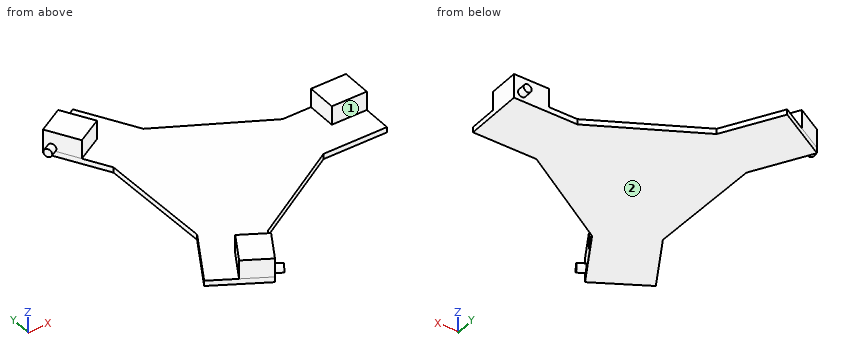
```python
from build123d import *

# Parameters (mm, degrees)
BOSS_EXTRUDE1_DEPTH = 2
SKETCH2_W           = 6.854235104
SKETCH2_H           = 13.064732657
BOSS_EXTRUDE2_DEPTH = 11
SKETCH3_W           = 13.064732657
SKETCH3_H           = 11
BOSS_EXTRUDE3_DEPTH = 7
SKETCH6_R           = 1.5
BOSS_EXTRUDE4_DEPTH = 3
SKETCH7_R           = 1.5
BOSS_EXTRUDE5_DEPTH = 3
SKETCH8_R           = 1.5
BOSS_EXTRUDE6_DEPTH = 3


with BuildPart() as part:
    # Sketch1 → Boss-Extrude1 (new body)
    with BuildSketch(Plane.XY):
        Polygon((30.93899215, 11.451445147), (54.645492629, 11.451445147), (54.645492629, -10.246029868), (30.93899215, -10.246029868), (-5.552253668, -32.519675743), (-17.405503908, -53.050107393), (-36.196068468, -42.201369885), (-24.342818229, -21.670938236), (-25.386738482, 21.068230596), (-37.239988722, 41.598662246), (-18.449424161, 52.447399753), (-6.596173922, 31.916968104), align=None)
    extrude(amount=BOSS_EXTRUDE1_DEPTH)

    # Sketch2 → Boss-Extrude2 (add)
    with BuildSketch(Plane(origin=(-9.917242407, -5.725722573, 0), x_dir=(0, 0, 1), z_dir=(-0.8660254037844431, -0.4999999999999922, 0))):
        with Locations((5.427117552, 48.1131263)):
            Rectangle(SKETCH2_W, SKETCH2_H)
    extrude(amount=-BOSS_EXTRUDE2_DEPTH)

    # Sketch3 → Boss-Extrude3 (add)
    with BuildSketch(Plane.XY.offset(2)):
        Polygon((-37.239988722, 41.598662246), (-27.71370928, 47.098662246), (-21.181342951, 35.784271871), (-30.707622393, 30.284271871), align=None)
        with Locations((48.1131263, 5.951445147)):
            Rectangle(SKETCH3_W, SKETCH3_H)
        Polygon((-10.873137579, -41.735717017), (-17.405503908, -53.050107393), (-26.931783349, -47.550107393), (-20.39941702, -36.235717017), align=None)
    extrude(amount=BOSS_EXTRUDE3_DEPTH)

    # Sketch6 → Boss-Extrude4 (add)
    with BuildSketch(Plane(origin=(-9.917242407, -5.725722573, 0), x_dir=(0, 0, 1), z_dir=(-0.8660254037844431, -0.4999999999999922, 0))):
        with Locations(Location((3, 51.645492629, 0), (0, 0, 270))):
            Circle(SKETCH6_R)
    extrude(amount=BOSS_EXTRUDE4_DEPTH)

    # Sketch7 → Boss-Extrude5 (add)
    with BuildSketch(Plane(origin=(9.917242407, -5.725722573, 0), x_dir=(0, 0, -1), z_dir=(0.8660254037844364, -0.5000000000000041, 0))):
        with Locations(Location((-3.057556163, -51.645492629, 0), (0, 0, 90))):
            Circle(SKETCH7_R)
    extrude(amount=BOSS_EXTRUDE5_DEPTH)

    # Sketch8 → Boss-Extrude6 (add)
    with BuildSketch(Plane(origin=(0, 11.451445147, 0), x_dir=(1, 0, 0), z_dir=(0, 1, 0))):
        with Locations(Location((51.645492629, -3, 0), (0, 0, 270))):
            Circle(SKETCH8_R)
    extrude(amount=BOSS_EXTRUDE6_DEPTH)


solid = part.part
```
Read the model definition and answer for the solid it produces. Units are mm, in the model's axes. Face numbers are marked on the shaded views. A direction names the side the tool comes from. Give positions to 0.01 mm unless a question says otherwise; leave off trailing zeros. Write each loop counter-clockwise with the first axis right and the second up, starting at its lowest first coordinate (ties: lowest second). Pieces come first, ordered by that corner, then holes. Notation, with made-up numbers: (43, 30) - (67, 30) arc R22 cw to (67, 36) - close; hole circle Ø8 at (52, 14.5). An arc over 180 degrees is marked (long way). Write item = value, one per line. Start each with the question number.
Item 1: Find section B-B (y = 27). Give the vertices of the cut face in (x, z).
Item 2: Each of these flat-tipped pins is pushed along its axis until it touches: P1, Ø5, axis at y = -42, z = 2, coming from the +X side; P2, Ø3.5, axis at x = 51, z = 3, coming from the +Y side; P3, Ø2, axis at x = 37, z = 0.5, coming from the -Y side; P4, Ø1, axis at y = 20.5, z = 3.5, coming from the -X side. Where does it stop, or does it pass through?
Item 3: Find section D-D (y = 10). Give the vertices of the cut face in (x, z), then the cut area to 3 significant figures.
Item 4: Find section A-A (z = 7.5). Give the vertices of the cut face in (x, y).
Item 5: Find the intervals of material crossed by probe 1 along Z at (x, y) = (6, 9.5); probe 2 along Y at (x, z) = (-14.5, 2.25); probe 3 along Y at (x, z) = (42, 6.5), in increasing order. Write a range as [from, to].
Item 6: Find section C-C (x = 25). Give the vertices of the cut face in (y, z), then the cut area to 3 significant figures.
Item 7: A tool of negligible diameter and unlimited length cuts with its end or side. For the marked faces 1 and 2, from which of +Z, -Z, +X, -X, +Y, -Y can it reach the whole face along a straight path? Write none if from no direction.
Response:
q1.outline = (-28.81, 0) - (2.42, 0) - (2.42, 2) - (-28.81, 2) - close
q2.P1 = -9.58
q2.P2 = 14.45
q2.P3 = -10.25
q2.P4 = through
q3.outline = (-25.12, 0) - (54.65, 0) - (54.65, 9) - (41.58, 9) - (41.58, 2) - (-25.12, 2) - close
q3.area = 251 mm²
q4.outline = (-37.24, 41.6) - (-30.71, 30.28) - (-21.18, 35.78) - (-27.71, 47.1) - close; (-26.93, -47.55) - (-17.41, -53.05) - (-10.87, -41.74) - (-20.4, -36.24) - close; (41.58, 0.45) - (54.65, 0.45) - (54.65, 11.45) - (41.58, 11.45) - close
q5.probe_1 = [0, 2]
q5.probe_2 = [-52.72, -49.8], [-48.02, -39.64]
q5.probe_3 = [0.45, 11.45]
q6.outline = (-13.87, 0) - (14.69, 0) - (14.69, 2) - (-13.87, 2) - close
q6.area = 57.1 mm²
q7.face_1 = +Z, +X, -X, -Y
q7.face_2 = -Z, +X, -X, +Y, -Y
